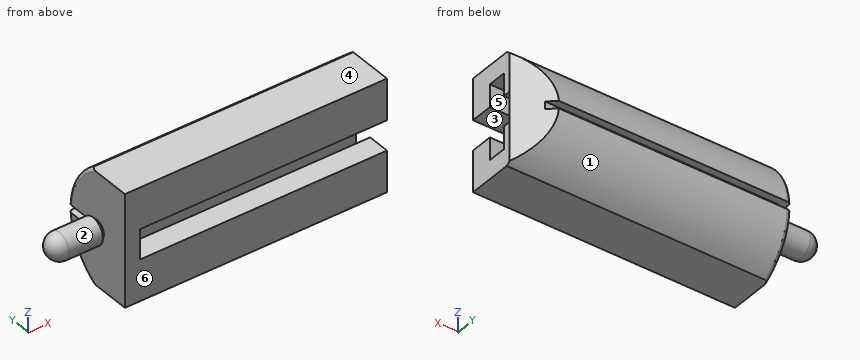
Autodesk Fusion 360 part; units mm, degrees
sketch "Sketch1" plane through (0, 0, 0) normal (0, 1, 0) x (1, 0, 0)
  line L0 (17.5, 7.5) -> (-17.5, 7.5)
  line L1 (-17.5, 7.5) -> (-17.5, -7.5)
  line L2 (-17.5, -7.5) -> (17.5, -7.5)
  line L3 (17.5, -7.5) -> (17.5, 7.5)
  line L4 (17.5, 7.5) -> (-17.5, -7.5) construction
  line L5 (-17.5, 7.5) -> (17.5, -7.5) construction
  dimension "d3" = 35
  dimension "d4" = 15
extrude "Extrude1" add sketch "Sketch1" along normal blind 10
sketch "Sketch2" plane through (17.5, 0, 0) normal (1, 0, 0) x (0, 0, -1)
  line L0 (-7.5, 0) -> (7.5, 0)
  line L1 (7.5, 0) -> (7.5, 10)
  line L2 (7.5, 10) -> (-7.5, 10)
  line L3 (-7.5, 10) -> (-7.5, 0)
  line L4 (-2, 0) -> (2, 0)
  line L5 (-2, 0) -> (-2, 3)
  line L6 (2, 0) -> (2, 3)
  line L7 (-2, 3) -> (-5, 3)
  line L8 (-5, 3) -> (-5, 5.5)
  line L9 (-5, 5.5) -> (-2, 5.5)
  line L10 (-2, 5.5) -> (-2, 6.5)
  line L11 (-2, 6.5) -> (2, 6.5)
  line L12 (2, 6.5) -> (2, 5.5)
  line L13 (2, 5.5) -> (5, 5.5)
  line L14 (5, 5.5) -> (5, 3)
  line L15 (5, 3) -> (2, 3)
  arc A0 (7.5, 6) -> (-7.5, 6) centre (0, 0.9687) ccw
  line L16 (-7.5, 6) -> (-7.5, 10)
  line L17 (7.5, 6) -> (7.5, 10)
  line L18 (7.5, 10) -> (-7.5, 10)
  dimension "d7" = 4
  dimension "d8" = 3
  dimension "d9" = 3
  dimension "d10" = 3
  dimension "d11" = 2.5
  dimension "d12" = 3
  dimension "d13" = 1
  dimension "d14" = 4
  dimension "d15" = 1
  dimension "d16" = 3
  dimension "d17" = 2.5
  dimension "d18" = 3
  dimension "d23" = 15
  dimension "d24" = 6
extrude "Extrude2" cut sketch "Sketch2" against normal blind 33 contours L0 L4 L5 L6 L7 L8 L9 L10 L11 L12 L13 L14 L15
extrude "Extrude3" cut sketch "Sketch2" against normal blind 35 contours L2 L3 A0 L16 L18 | L1 L2 A0 L17 L18
sketch "Sketch3" plane through (0, 0, 0) normal (0, 0, 1) x (1, 0, 0)
  line L0 (17.5, 6.5) -> (13.5, 10)
  line L1 (13.5, 10) -> (17.5, 10)
  line L2 (17.5, 10) -> (17.5, 6.5)
  point P0 (17.5, 0)
  dimension "d28" = 6.5
extrude "Extrude4" cut sketch "Sketch3" along normal blind 7.5 and the other way blind 7.5
fillet "Fillet1" radius 0.5 1 edges at (-17.5, 10, 0)
sketch "Sketch4" plane through (-17.5, 0, 0) normal (-1, 0, 0) x (0, 0, 1)
  arc A0 (7.5, 5.0347) -> (-7.5, 5.0347) centre (0, 0.9688) ccw
  line L0 (-7.5, 5.0347) -> (-7.5, 0)
  line L1 (-7.5, 0) -> (7.5, 0)
  line L2 (7.5, 0) -> (7.5, 5.0347)
  circle A1 centre (0, 5) radius 1.75
  circle A2 centre (0, 5) radius 1.25
  dimension "d36" = 3.5
  dimension "d38" = 2.5
extrude "Extrude5" add sketch "Sketch4" along normal blind 5 contours A1 | A2
extrude "Extrude6" cut sketch "Sketch4" along normal blind 0.5 contours A1
sketch "Sketch6" plane through (0, 0, 0) normal (0, 0, 1) x (1, 0, 0)
  line L0 (-22.5, 6.75) -> (-22.5, 5)
  line L1 (-22.5, 5) -> (-24.25, 5)
  arc A0 (-22.5, 6.75) -> (-24.25, 5) centre (-22.5, 5) ccw
  dimension "d46" = 1.75
revolve "Revolve1" add sketch "Sketch6" angle 360 about axis through (-22.5, 5, 0) along (-1, 0, 0)
sketch "Sketch7" plane through (-17.5, 0, 0) normal (-1, 0, 0) x (0, 0, 1)
  circle A0 centre (0, 5) radius 1.25
  arc A1 (7.5, 5.0347) -> (-7.5, 5.0347) centre (0, 0.9688) ccw
  line L0 (-7.5, 5.0347) -> (-7.5, 0)
  line L1 (-7.5, 0) -> (7.5, 0)
  line L2 (7.5, 0) -> (7.5, 5.0347)
  line L3 (-0.5, 10) -> (-0.5, 5)
  line L4 (-0.5, 10) -> (0.5, 10)
  line L5 (0.5, 10) -> (0.5, 5)
  line L6 (-0.5, 5) -> (0.5, 5)
  dimension "d48" = 1
  dimension "d49" = 5
extrude "Extrude7" cut sketch "Sketch7" against normal blind 1 contours A0 L3 L5 L6 | A0 A1 L3 L5 | A1 L3 L4 L5 picked at (-0.0252, 4.5841)
sketch "Sketch8" plane through (-16.5, 0, 0) normal (-1, 0, 0) x (0, 0, 1)
  arc A0 (0.5, 9.9861) -> (-0.5, 9.9861) centre (0, 0.9687) ccw
  line L0 (-0.5, 9.9861) -> (-0.5, 5)
  line L1 (-0.5, 5) -> (0.5, 5)
  line L2 (0.5, 5) -> (0.5, 9.9861)
  line L3 (-0.5, 10) -> (0.5, 10)
  line L4 (0.5, 10) -> (0.5, 9)
  line L5 (0.5, 9) -> (-0.5, 9)
  line L6 (-0.5, 9) -> (-0.5, 10)
extrude "Extrude8" cut sketch "Sketch8" against normal blind 35 contours A0 L0 L2 L4 L5 L6
Read the model definition and answer for the solid it produces. Units are mm, in the model's axes. Face numbers are marked on the shaded views. A direction names the side the tool comes from. Give positions to 0.01 mm unless a question says otherwise; leave off trailing zeros. Order: outer loops, then holes, each group sorted by start corner. A loop starts at its lowest first (then second) coordinate and runs counter-clockwise, first axis right, second up. Notation, with made-up numbers: (33, 1.25) -> (68, 1.25) arc R13 ccw to (68, 19.25) -> close; hole circle Ø8 at (31.5, -5). An arc over 180 degrees is marked (long way). Write item = value, one per line.
1. The mould has two halves that part along Y. Classify the marked faces 4, 5 and 6: +Y half, -Y half, draft (parallel to the pull), parting line (faces both ways), or undercut.
Numbers:
face_4 = draft
face_5 = undercut
face_6 = -Y half
2. A cutting plane is placed at B-B, the plane y = 1. Write down the section's boundary in (x, z), and give its area (3 significant figures).
Numbers:
outline = (-17.5, -7.5) -> (17.5, -7.5) -> (17.5, -2) -> (-15.5, -2) -> (-15.5, 2) -> (17.5, 2) -> (17.5, 7.5) -> (-17.5, 7.5) -> close
area = 393 mm²
3. A cutting plane is placed at A-A, the plane z = 0. Write down the section's boundary in (x, y), and give its area (3 significant figures).
Numbers:
outline = (-22.5, 3.25) -> (-18, 3.25) -> (-18, 3.75) -> (-17.5, 3.75) -> (-17.5, 0) -> (-15.5, 0) -> (-15.5, 6.5) -> (17.5, 6.5) -> (14.64, 9) -> (-16.5, 9) -> (-16.5, 6.25) -> (-18, 6.25) -> (-18, 6.75) -> (-22.5, 6.75) arc R1.75 ccw to start; hole (-17.5, 3.75) -> (-16.5, 3.75) -> (-16.5, 5) -> (-17.5, 5) -> close
area = 115 mm²
4. Given pin 1 (5 mm diameter, centred on y = 7, z = -3, fed in from +X); pin 2 (1.9 mm diameter, centred on x = -7, y = 8, fed in from +Z); pin 3 (0.5 mm diameter, centred on y = 8.5, z = 0, fed in from -X); pin 4 (1 mm diameter, centred on y = 5.5, z = -0.5, fed in from +X), each flat-ended and moving along its own axis, determine where each tip first touches the part or whether it passes through.
Numbers:
pin_1 = 17.5
pin_2 = 6.68
pin_3 = -16.5
pin_4 = -15.5
5. For the marked faces 1, 2 and 3, determine the directions among +Z, -Z, +X, -X, +Y, -Y from which every point of the face is accessible in a straight line to the end or side of a thin tool.
Numbers:
face_1 = -Z, +X, -X, +Y
face_2 = -X
face_3 = +X, -Y
6. Straight lines are drawn through the part: line 1 along Y through (x, z) = (-17.15, 0); line 2 along Z through (x, y) = (-8.5, 1); line 3 along Z through (x, y) = (-3, 4). For each, find the intervals that lie inside material, in ascending order.
Numbers:
line_1 = 0 to 3.75, 5 to 6.25
line_2 = -7.5 to -2, 2 to 7.5
line_3 = -7.5 to -5, 5 to 7.5
7. A cutting plane is placed at D-D, the plane x = -19. Write down the section's boundary in (y, z).
Numbers:
outline = circle Ø3.5 at (5, 0)
